from build123d import *

# Parameters (mm, degrees)
SKETCH1_W                      = 203.2
SKETCH1_H                      = 34.925
BOSS_EXTRUDE1_DEPTH            = 6.35
BOSS_EXTRUDE3_START            = 19.05
SKETCH2_W                      = 203.2
SKETCH2_H                      = 101.6
BOSS_EXTRUDE3_DEPTH            = 3.175
BOSS_EXTRUDE4_REACH            = 117.746
SKETCH3_W                      = 6.35
SKETCH3_H                      = 6.35
SKETCH4_W                      = 76.2
SKETCH4_H                      = 6.35
CUT_EXTRUDE1_DEPTH             = 3.175
BOSS_EXTRUDE5_START            = -190.5
SKETCH5_W                      = 3.175
SKETCH5_H                      = 3.175
BOSS_EXTRUDE5_DEPTH            = 3.175
F_2_CLEARANCE_HOLE1_D          = 2.4384
FILLET1_R                      = 15.875
FILLET2_R                      = 6.35
F_4_40_TAPPED_HOLE2_D          = 2.2606
SKETCH15_R                     = 3.175
BOSS_EXTRUDE6_DEPTH            = 1.5875
SKETCH20_W                     = 1.63195
SKETCH20_H                     = 25.4
F_4_CLEARANCE_HOLE3_AT_2_COUNT = 2
F_4_CLEARANCE_HOLE3_AT_2_PITCH = 18.25625
F_4_CLEARANCE_HOLE3_AT_3_COUNT = 2
F_4_CLEARANCE_HOLE3_AT_3_PITCH = 63.787085414
F_4_CLEARANCE_HOLE3_AT_4_COUNT = 2
F_4_CLEARANCE_HOLE3_AT_4_PITCH = 61.11875
BOSS_EXTRUDE11_DEPTH           = 4.318
FILLET10_RADIUS                = 1.5875
FILLET10_LENGTH                = 4.318
FILLET11_RADIUS                = 1.5875
FILLET11_LENGTH                = 4.318
FILLET12_R                     = 3.175
FILLET14_R                     = 15.875
SKETCH23_R                     = 3.175
BOSS_EXTRUDE12_DEPTH           = 3.175
CUT_EXTRUDE2_REACH             = 121.852
SKETCH26_W                     = 25.4
SKETCH26_H                     = 12.7
F_4_40_TAPPED_HOLE3_D          = 2.2606
F_4_40_TAPPED_HOLE3_DEPTH      = 6.35


with BuildPart() as part:
    # Sketch1 → Boss-Extrude1 (new body)
    with BuildSketch(Plane(origin=(0, 0, 0), x_dir=(1, 0, 0), z_dir=(0, 1, 0))):
        Rectangle(SKETCH1_W, SKETCH1_H)
    extrude(amount=BOSS_EXTRUDE1_DEPTH)


with BuildPart() as body_2:
    # Sketch2 → Boss-Extrude3 (new body)
    with BuildSketch(Plane(origin=(0, 6.35, 0), x_dir=(1, 0, 0), z_dir=(0, 1, 0)).offset(BOSS_EXTRUDE3_START)):
        Rectangle(SKETCH2_W, SKETCH2_H)
    extrude(amount=BOSS_EXTRUDE3_DEPTH)

    # Sketch3 → Boss-Extrude4 (add, up to next)
    with BuildSketch(Plane(origin=(0, 6.35, 0), x_dir=(1, 0, 0), z_dir=(0, 1, 0)), mode=Mode.PRIVATE) as boss_extrude4_sk1:
        with Locations((98.425, -14.2875)):
            Rectangle(SKETCH3_W, SKETCH3_H)
    boss_extrude4_tool1 = extrude(boss_extrude4_sk1.sketch, amount=BOSS_EXTRUDE4_REACH, mode=Mode.PRIVATE) - body_2.part
    # Sketch3 → Boss-Extrude4 (add, up to next)
    with BuildSketch(Plane(origin=(0, 6.35, 0), x_dir=(1, 0, 0), z_dir=(0, 1, 0)), mode=Mode.PRIVATE) as boss_extrude4_sk2:
        with Locations((98.425, 14.2875)):
            Rectangle(SKETCH3_W, SKETCH3_H)
    boss_extrude4_tool2 = extrude(boss_extrude4_sk2.sketch, amount=BOSS_EXTRUDE4_REACH, mode=Mode.PRIVATE) - body_2.part

    add(part.part)  # Boss-Extrude4 merges part
    add(boss_extrude4_tool1.solids().sort_by_distance((98.425, 6.35, 14.2875))[0])
    add(boss_extrude4_tool2.solids().sort_by_distance((98.425, 6.35, -14.2875))[0])

    # Sketch4 → Cut-Extrude1 (cut)
    with BuildSketch(Plane(origin=(0, 28.575, 0), x_dir=(1, 0, 0), z_dir=(0, 1, 0))):
        with Locations((-63.5, -26.9875)):
            Rectangle(SKETCH4_W, SKETCH4_H)
        with Locations((-63.5, 26.9875)):
            Rectangle(SKETCH4_W, SKETCH4_H)
    extrude(amount=-CUT_EXTRUDE1_DEPTH, mode=Mode.SUBTRACT)

    # Sketch5 → Boss-Extrude5 (add)
    with BuildSketch(Plane(origin=(101.6, 0, 0), x_dir=(0, 0, -1), z_dir=(1, 0, 0)).offset(BOSS_EXTRUDE5_START)):
        with Locations((-44.45, 23.8125)):
            Rectangle(SKETCH5_W, SKETCH5_H)
        with Locations((44.45, 23.8125)):
            Rectangle(SKETCH5_W, SKETCH5_H)
    extrude(amount=-BOSS_EXTRUDE5_DEPTH)

    # #2 Clearance Hole1 (through all)
    with Locations(Plane(origin=(0, 25.4, 0), x_dir=(-1, 0, 0), z_dir=(0, -1, 0))):
        with Locations((88.9, 33.147), (88.9, -33.147)):
            Hole(F_2_CLEARANCE_HOLE1_D / 2)

    # Fillet1
    fillet1_edges = [body_2.edges().sort_by_distance(p)[0] for p in [
        (101.6, 26.9875, 50.8),
        (101.6, 26.9875, -50.8),
    ]]
    fillet(fillet1_edges, radius=FILLET1_R)

    # Fillet2
    fillet2_edges = [body_2.edges().sort_by_distance(p)[0] for p in [
        (95.25, 6.35, 14.2875),
        (95.25, 6.35, -14.2875),
        (101.6, 0, 0),
    ]]
    fillet(fillet2_edges, radius=FILLET2_R - 0.0001)  # a hair under: the kernel refuses the full size

    # #4-40 Tapped Hole2 (through all)
    with Locations(Plane(origin=(0, 25.4, 0), x_dir=(-1, 0, 0), z_dir=(0, -1, 0))):
        with Locations((-87.3125, -44.45), (-87.3125, -26.19375), (-26.19375, -26.19375), (-26.19375, -44.45)):
            Hole(F_4_40_TAPPED_HOLE2_D / 2)

    # Sketch15 → Boss-Extrude6 (add)
    with BuildSketch(Plane.XZ.offset(-25.4)):
        with Locations(Location((26.19375, 44.45, 0), (0, 0, 270))):
            Circle(SKETCH15_R)
        with Locations(Location((87.3125, 44.45, 0), (0, 0, 270))):
            Circle(SKETCH15_R)
        with Locations(Location((87.3125, 26.19375, 0), (0, 0, 270))):
            Circle(SKETCH15_R)
        with Locations(Location((26.19375, 26.19375, 0), (0, 0, 270))):
            Circle(SKETCH15_R)
    extrude(amount=BOSS_EXTRUDE6_DEPTH)

    # Sketch20 → #4 Clearance Hole3 (revolve, cut)
    with BuildSketch(Plane(origin=(87.3125, 25.4, 44.45), x_dir=(0, 0, 1), z_dir=(1, 0, 0))):
        with Locations((0.815975, 12.7)):
            Rectangle(SKETCH20_W, SKETCH20_H)
    f_4_clearance_hole3 = revolve(axis=Axis((87.3125, 31.75, 44.45), (0, -1, 0)), mode=Mode.SUBTRACT)

    # #4 Clearance Hole3 at 2: #4 Clearance Hole3 ×2
    with Locations(*[(0, 0, -i * F_4_CLEARANCE_HOLE3_AT_2_PITCH) for i in range(1, F_4_CLEARANCE_HOLE3_AT_2_COUNT)]):
        add(f_4_clearance_hole3, mode=Mode.SUBTRACT)

    # #4 Clearance Hole3 at 3: #4 Clearance Hole3 ×2
    with Locations(*[Vector(-0.9581680931685116, 0, -0.28620605380358144) * (i * F_4_CLEARANCE_HOLE3_AT_3_PITCH) for i in range(1, F_4_CLEARANCE_HOLE3_AT_3_COUNT)]):
        add(f_4_clearance_hole3, mode=Mode.SUBTRACT)

    # #4 Clearance Hole3 at 4: #4 Clearance Hole3 ×2
    with Locations(*[(-i * F_4_CLEARANCE_HOLE3_AT_4_PITCH, 0, 0) for i in range(1, F_4_CLEARANCE_HOLE3_AT_4_COUNT)]):
        add(f_4_clearance_hole3, mode=Mode.SUBTRACT)

    # Sketch22 → Boss-Extrude11 (add)
    with BuildSketch(Plane.ZY.offset(101.6)):
        Polygon((17.065625, 0), (12.747625, 0), (12.747625, -6.477), (7.985125, -6.477), (7.985125, -9.652), (17.065625, -9.652), align=None)
        Polygon((-7.985125, -6.477), (-12.747625, -6.477), (-12.747625, 0), (-17.065625, 0), (-17.065625, -9.652), (-7.985125, -9.652), align=None)
    extrude(amount=-BOSS_EXTRUDE11_DEPTH)

    # Fillet10: full round fillet: the end face becomes a half cylinder, R = half its width
    fillet10_face = Plane((-99.441, -8.0645, 7.985125), x_dir=(-1, 0, 0), z_dir=(0, 0, -1))  # on the end face: x along it, z out of the body
    fillet10_slab = fillet10_face.offset(-FILLET10_RADIUS / 2) * Box(FILLET10_LENGTH, 2 * FILLET10_RADIUS, FILLET10_RADIUS, mode=Mode.PRIVATE)  # the body's end, R deep
    fillet10_round = Plane((-99.441, -8.0645, 9.572625), x_dir=(0, 0, -1), z_dir=(-1, 0, 0)) * Cylinder(FILLET10_RADIUS, FILLET10_LENGTH, mode=Mode.PRIVATE)  # its axis R under the face
    add(fillet10_slab - fillet10_round, mode=Mode.SUBTRACT)

    # Fillet11: full round fillet: the end face becomes a half cylinder, R = half its width
    fillet11_face = Plane((-99.441, -8.0645, -7.985125), x_dir=(-1, 0, 0), z_dir=(0, 0, 1))  # on the end face: x along it, z out of the body
    fillet11_slab = fillet11_face.offset(-FILLET11_RADIUS / 2) * Box(FILLET11_LENGTH, 2 * FILLET11_RADIUS, FILLET11_RADIUS, mode=Mode.PRIVATE)  # the body's end, R deep
    fillet11_round = Plane((-99.441, -8.0645, -9.572625), x_dir=(0, 0, 1), z_dir=(-1, 0, 0)) * Cylinder(FILLET11_RADIUS, FILLET11_LENGTH, mode=Mode.PRIVATE)  # its axis R under the face
    add(fillet11_slab - fillet11_round, mode=Mode.SUBTRACT)

    # Fillet12
    fillet12_edges = [body_2.edges().sort_by_distance(p)[0] for p in [
        (-99.441, -9.652, 17.065625),
        (-99.441, -9.652, -17.065625),
    ]]
    fillet(fillet12_edges, radius=FILLET12_R)

    # Fillet14
    fillet14_edges = [body_2.edges().sort_by_distance(p)[0] for p in [
        (-101.6, 26.9875, -50.8),
        (-101.6, 26.9875, 50.8),
    ]]
    fillet(fillet14_edges, radius=FILLET14_R)

    # Sketch23 → Boss-Extrude12 (add)
    with BuildSketch(Plane(origin=(0, 28.575, 0), x_dir=(1, 0, 0), z_dir=(0, 1, 0))):
        with Locations(Location((3.175, 12.7, 0), (0, 0, 90))):
            Circle(SKETCH23_R)
        with Locations(Location((3.175, 47.625, 0), (0, 0, 90))):
            Circle(SKETCH23_R)
        with Locations(Location((82.55, 12.7, 0), (0, 0, 90))):
            Circle(SKETCH23_R)
        with Locations(Location((82.55, 47.625, 0), (0, 0, 90))):
            Circle(SKETCH23_R)
    extrude(amount=BOSS_EXTRUDE12_DEPTH)

    # Sketch26 → Cut-Extrude2 (cut, up to next)
    with BuildSketch(Plane(origin=(0, 28.575, 0), x_dir=(1, 0, 0), z_dir=(0, 1, 0)), mode=Mode.PRIVATE) as cut_extrude2_sk1:
        Rectangle(SKETCH26_W, SKETCH26_H)
    cut_extrude2_tool1 = extrude(cut_extrude2_sk1.sketch, amount=-CUT_EXTRUDE2_REACH, mode=Mode.PRIVATE) & body_2.part
    add(cut_extrude2_tool1.solids().sort_by_distance((0, 28.575, 0))[0], mode=Mode.SUBTRACT)

    # #4-40 Tapped Hole3
    with Locations(Plane(origin=(0, 31.75, 0), x_dir=(1, 0, 0), z_dir=(0, 1, 0))):
        with Locations((3.175, 47.625), (3.175, 12.7), (82.55, 12.7), (82.55, 47.625)):
            Hole(F_4_40_TAPPED_HOLE3_D / 2, depth=F_4_40_TAPPED_HOLE3_DEPTH)


solid = body_2.part
Work out the finished part from the listing and answer in its coordinate system (mm). A direction names the side the tool comes from. Round coordinates to 2 decimals unless told otherwise and drop trailing zeros. Write each loop counter-clockwise with the first axis right and the second up, starting at its lowest first coordinate (ties: lowest second). Pieces come first, ordered by that corner, then holes. Notation, with made-up numbers: (24, 30) -> (28, 30) arc R23 cw to (28, 59) -> close; hole circle Ø4 at (22, 20.25). An arc over 180 degrees is marked (long way). Answer as CSV lines item,"result". Start each with the question number.
(1) A tool of negligible diameter and unlimited length cuts with its end or side. For faces 4 (the cylindrical face through (89.99, 24.62, 42.74)), 5 (the flat face through (95.25, 19, -14)), 6 (the flat face through (98, 16, -11.112)), from which of +Z, -Z, +X, -X, +Y, -Y can it reach the whole face along a straight path? Write none if from no direction.
(2) Each of these flat-tipped pins is pushed along its axis until it touches: pin 1 (4 mm diameter, centred on x = 26.19, z = 44.45, fed in from -Y); pin 2 (12 mm diameter, centred on x = -12, y = 5, fed in from -Z); pin 3 (2 mm diameter, centred on x = 87.31, z = 26.19, fed in from -Y); pin 4 (3 mm diameter, centred on x = 87.31, z = 26.19, fed in from -Y). Where does it stop, or does it pass through?
(3) Find the intervals of material crossed by probe 1 along Z at (x, y) = (82.55, 27.25); probe 2 along X at (y, z) = (25, 43) (3 decimals); probe 3 along Y at (x, z) = (63.5, 16) (3 decimals), in increasing order.
(4) The mould has two halves that part along X. Classify faces 1 (the cylindrical face through (5.107, 30.14, -10.18)), 2 (the flat face through (95.25, 19, 14)), 3 (the flat face through (-99, -3, -12.748)): +X half, -X half, draft (parallel to the pull), parting line (faces both ways), or undercut.
(5) The part is cut by section B-B, the plane y = 15. Give the vertices of the cut face in (x, z), then the cut area to 3 significant figures.
(6) The part is cut by section A-A, the plane x = -51.5. Give the number of separate pieces and of enclosed holes in the cut face, then the cut area to 3 significant figures.
Output values:
1,face 4,"-Y"
1,face 5,"+Z, -Z, -X"
1,face 6,"+X, -X"
2,pin 1,"stops at y = 23.81"
2,pin 2,"stops at z = -17.46"
2,pin 3,"passes through"
2,pin 4,"stops at y = 25.4"
3,probe 1,"z = -50.8 to -48.76, -46.49 to -13.83, -11.57 to 50.8"
3,probe 2,"x = -92.075 to -88.9, 23.369 to 25.445, 26.943 to 29.018, 84.488 to 86.564, 88.061 to 90.137"
3,probe 3,"y = 0 to 6.35, 25.4 to 28.575"
4,face 1,"undercut"
4,face 2,"-X half"
4,face 3,"draft"
5,outline,"(95.25, -17.46) -> (101.6, -17.46) -> (101.6, -11.11) -> (95.25, -11.11) -> close; (95.25, 11.11) -> (101.6, 11.11) -> (101.6, 17.46) -> (95.25, 17.46) -> close"
5,area,"80.6 mm²"
6,separate pieces,"4"
6,enclosed holes,"0"
6,area,"504 mm²"
